from build123d import *

# Parameters (mm, degrees)
SKETCH1_R          = 6.3
EXTRUDE1_DEPTH     = 127
SKETCH2_R          = 7.486213626
EXTRUDE2_DEPTH     = 10.18
FILLET1_R          = 1.27
CUT_EXTRUDE1_DEPTH = 10.18
LPATTERN1_COUNT    = 13
LPATTERN1_PITCH    = 1.74


with BuildPart() as part:
    # Sketch1 → Extrude1 (new body)
    with BuildSketch(Plane.XY):
        Circle(SKETCH1_R)
    extrude(amount=EXTRUDE1_DEPTH)

    # Sketch2 → Extrude2 (add)
    with BuildSketch(Plane.XY.offset(127)):
        Circle(SKETCH2_R)
    extrude(amount=EXTRUDE2_DEPTH)

    # Fillet1
    fillet1_edges = [part.edges().sort_by_distance(p)[0] for p in [
        (-7.486213626, 0, 137.18),
    ]]
    fillet(fillet1_edges, radius=FILLET1_R)

    # Sketch3 → Cut-Extrude1 (cut)
    with BuildSketch(Plane.XY.offset(137.18)):
        Polygon((4.202603037, 2.423907976), (0.002135635, 4.85151498), (-4.200467402, 2.427607004), (-4.202603037, -2.423907976), (-0.002135635, -4.85151498), (4.200467402, -2.427607004), align=None)
    extrude(amount=-CUT_EXTRUDE1_DEPTH, mode=Mode.SUBTRACT)

    # Sketch4 → Cut-Revolve1 (revolve, cut)
    with BuildSketch(Plane(origin=(0, 0, 0), x_dir=(1, 0, 0), z_dir=(0, 1, 0))):
        Polygon((-6.3, 0), (-5.861323423, -0.438676577), (-6.3, -0.877353155), (-6.738676577, -0.438676577), align=None)
    cut_revolve1 = revolve(axis=Axis((0, 0, 127), (0, 0, -1)), mode=Mode.SUBTRACT)

    # LPattern1: Cut-Revolve1 ×13
    with Locations(*[(0, 0, i * LPATTERN1_PITCH) for i in range(1, LPATTERN1_COUNT)]):
        add(cut_revolve1, mode=Mode.SUBTRACT)


solid = part.part
Could you check a few things on this model? Use its own coordinates, in mm. A direction names the side the tool comes from. Coordinates: 2 decimals unless noted, no trailing zeros. Order: outer loops, then holes, each group sorted by start corner. A loop starts at its lowest first (then second) coordinate and runs counter-clockwise, first axis right, second up. Notation, with made-up numbers: (-30, -39.5) -> (-21, -39.5) arc R16 ccw to (-21, -29.5) -> close; hole circle Ø2 at (21, 36). An arc over 180 degrees is marked (long way). One line per item, written item: value. Start each with the question number.
1) Imagine slicing it at A-A on z = 56. List the corners of the cut face in (x, y) for me, plus the area to 3 significant figures.
2) If I drill on L1, parallel to X at y = 4, z = 26.5; L2, parallel to Z at x = -2.5, y = -3.25; L3, parallel to Y at x = 0, z = 17, over which ranges is the centre line in solid material (lowest first)? Write a range as [from, to].
3) Which directions (+Z, -Z, +X, -X, +Y, -Y) give clear straight access to the entire face, cutting with the end or side of a thin tool? Please do faces 1 (the cylindrical face through (-5, -3.83, 73.64)), 2 (the flat face through (-2.13, -3.62, 132.16)).
4) I'm going to push flat-ended pins straight in: pin 1 (1.5 mm diameter, centred on y = 2.5, z = 81.5, fed in from -X); pin 2 (3 mm diameter, centred on y = 4, z = 100, fed in from +X). Where does each tip first touch, or does it pass through?
Answer list:
1. outline: circle Ø12.6 at (0, 0)
1. area: 125 mm2
2. L1: x = [-4.87, 4.87]
2. L2: z = [0, 127]
2. L3: y = [-6.3, 6.3]
3. face 1: -Z
3. face 2: +Z
4. pin 1: stops at x = -6.05
4. pin 2: stops at x = 5.78
